Check sheet for the modelled part. Datum: model origin and axes. Units: mm. A direction names the side the tool comes from. Coordinates: 2 decimals unless noted, no trailing zeros. Loops run counter-clockwise (first coordinate to the right, second up) from the corner with the lowest first, then second, coordinate; pieces in that order, holes last. Notation, with made-up numbers: (8, -30) - (64, -30) arc R31 cw to (64, 7) - close; hole circle Ø2 at (-23.75, 36). An arc over 180 degrees is marked (long way). Write each question's results on one line, items separated by ' | '. Start each with the question number.
1. Thickness scan on line 1 (Y direction, x = 0, z = -0.5) (3 decimals); line 2 (Y direction, x = -21.5, z = 0); line 3 (X direction, y = -12.5, z = -0.1). Record the ranges inside material, lowest first. Write a range as [from, to].
2. Cross-section at A-A (x = 0). Record the cut outline in (y, z) (3 decimals), and give its area (3 significant figures).
3. Tool access check on faces 5 (the face through (29.563, 7.238, 0.268)), 6 (the face through (16.02, -25.88, 0.27)), 7 (the face through (-20.35, -15.655, 0.268)). Record the directions out of +Z, -Z, +X, -X, +Y, -Y that give a thin tool (end or side, any length) a straight path to the whole face; none if there is none.
4. Cross-section at D-D (y = -13). Record the cut outline in (x, z), and give its area (3 significant figures).
5. Cross-section at C-C (y = 0). Record the cut outline in (x, z) (3 decimals), and give its area (3 significant figures).
6. Cross-section at B-B (z = 1.05). Record the cut outline in (x, y) (3 decimals).
7. Draft check along Y on faces 1 (the face through (2, 1, 0)), 2 (the face through (-27.469, -12.837, 0.268)), 3 (the face through (-19.66, -23.23, 0.27)), 4 (the face through (-11.646, 32.475, 0.268)). Enter one of: released by +Y, released by -Y, zero draft, split by the parting line, or undercut.
8. Gauge pin test, flat end, axial feed: P1, Ø2.5, axis at x = -0.5, y = -1, coming from the -Z side. Record the tip position at first contact, or that the pin passes through.
```python
from build123d import *

# Parameters (mm, degrees)
BOSS_EXTRUDE1_DEPTH = 1.5
SKETCH2_R           = 4.075
BOSS_EXTRUDE2_DEPTH = 1
SKETCH3_R           = 2
CUT_EXTRUDE1_DEPTH  = 2.5


with BuildPart() as part:
    # Sketch1 → Boss-Extrude1 (new body)
    with BuildSketch(Plane.XY):
        with BuildLine():
            Line((-23.460220375, 25.295613453), (-18.010816917, 19.106590755))
            Line((-18.010816917, 19.106590755), (-24.257098112, 10.052090702))
            Line((-24.257098112, 10.052090702), (-31.977876551, 12.948567925))
            ThreePointArc((-31.977876551, 12.948567925), (-34.489701397, -0.842910146), (-31.307164796, -14.495221021))
            Line((-31.307164796, -14.495221021), (-23.737096152, -11.225043545))
            Line((-23.737096152, -11.225043545), (-17.055961915, -19.96360437))
            Line((-17.055961915, -19.96360437), (-22.1965272, -26.411440329))
            ThreePointArc((-22.1965272, -26.411440329), (-9.856248675, -33.062128819), (4.11132844, -34.254152718))
            Line((4.11132844, -34.254152718), (3.340484701, -26.044049191))
            Line((3.340484701, -26.044049191), (13.715933938, -22.39027674))
            Line((13.715933938, -22.39027674), (18.259668309, -29.27173574))
            ThreePointArc((18.259668309, -29.27173574), (28.398204714, -19.590609204), (33.84810551, -6.675009615))
            Line((33.84810551, -6.675009615), (25.801629236, -4.87106406))
            Line((25.801629236, -4.87106406), (25.532875276, 6.125652327))
            Line((25.532875276, 6.125652327), (33.481622838, 8.320512732))
            ThreePointArc((33.481622838, 8.320512732), (27.407304408, 20.95446647), (16.80795122, 30.128769901))
            Line((16.80795122, 30.128769901), (12.605799132, 23.03356604))
            Line((12.605799132, 23.03356604), (2.064250813, 26.176138082))
            Line((2.064250813, 26.176138082), (2.433112603, 34.414095412))
            ThreePointArc((2.433112603, 34.414095412), (-11.45955905, 32.541181699), (-23.460220375, 25.295613453))
        make_face()
    extrude(amount=BOSS_EXTRUDE1_DEPTH)

    # Sketch2 → Boss-Extrude2 (add)
    with BuildSketch(Plane(origin=(0, 0, 0), x_dir=(-1, 0, 0), z_dir=(0, 0, -1))):
        with BuildLine():
            Line((-2.433112603, 34.414095412), (-2.064250813, 26.176138082))
            Line((-2.064250813, 26.176138082), (-12.605799132, 23.03356604))
            Line((-12.605799132, 23.03356604), (-16.80795122, 30.128769901))
            ThreePointArc((-16.80795122, 30.128769901), (-27.407304408, 20.95446647), (-33.481622838, 8.320512732))
            Line((-33.481622838, 8.320512732), (-25.532875276, 6.125652327))
            Line((-25.532875276, 6.125652327), (-25.801629236, -4.87106406))
            Line((-25.801629236, -4.87106406), (-33.84810551, -6.675009615))
            ThreePointArc((-33.84810551, -6.675009615), (-28.398204714, -19.590609204), (-18.259668309, -29.27173574))
            Line((-18.259668309, -29.27173574), (-13.715933938, -22.39027674))
            Line((-13.715933938, -22.39027674), (-3.340484701, -26.044049191))
            Line((-3.340484701, -26.044049191), (-4.11132844, -34.254152718))
            ThreePointArc((-4.11132844, -34.254152718), (9.856248675, -33.062128819), (22.1965272, -26.411440329))
            Line((22.1965272, -26.411440329), (17.055961915, -19.96360437))
            Line((17.055961915, -19.96360437), (23.737096152, -11.225043545))
            Line((23.737096152, -11.225043545), (31.307164796, -14.495221021))
            ThreePointArc((31.307164796, -14.495221021), (34.489701397, -0.842910146), (31.977876551, 12.948567925))
            Line((31.977876551, 12.948567925), (24.257098112, 10.052090702))
            Line((24.257098112, 10.052090702), (18.010816917, 19.106590755))
            Line((18.010816917, 19.106590755), (23.460220375, 25.295613453))
            ThreePointArc((23.460220375, 25.295613453), (11.45955905, 32.541181699), (-2.433112603, 34.414095412))
        make_face()
        Circle(SKETCH2_R, mode=Mode.SUBTRACT)
    extrude(amount=BOSS_EXTRUDE2_DEPTH)

    # Sketch3 → Cut-Extrude1 (cut, through all)
    with BuildSketch(Plane(origin=(0, 0, 0), x_dir=(-1, 0, 0), z_dir=(0, 0, -1))):
        Circle(SKETCH3_R)
    extrude(amount=-CUT_EXTRUDE1_DEPTH, mode=Mode.SUBTRACT)


solid = part.part
```
Established:
1) line 1: [-34.5, -4.075], [4.075, 34.5] | line 2: [-26.98, -25.54], [-14.15, 14.05], [23.07, 26.98] | line 3: [-32.16, -26.69], [-22.76, 32.16]
2) outline: (-34.5, -1) - (-4.075, -1) - (-4.075, 0) - (-2, 0) - (-2, 1.5) - (-34.5, 1.5) - close; (2, 0) - (4.075, 0) - (4.075, -1) - (34.5, -1) - (34.5, 1.5) - (2, 1.5) - close | area: 158 mm^2
3) face 5: +Z, -Z, +X | face 6: +Z, -Z, -Y | face 7: +Z, -Z
4) outline: (-31.96, -1) - (-27.85, -1) - (-27.85, 1.5) - (-31.96, 1.5) - close; (-22.38, -1) - (31.96, -1) - (31.96, 1.5) - (-22.38, 1.5) - close | area: 146 mm^2
5) outline: (-34.5, -1) - (-4.075, -1) - (-4.075, 0) - (-2, 0) - (-2, 1.5) - (-34.5, 1.5) - close; (2, 0) - (4.075, 0) - (4.075, -1) - (25.683, -1) - (25.683, 1.5) - (2, 1.5) - close | area: 136 mm^2
6) outline: (-31.978, 12.949) arc R34.5 ccw to (-31.307, -14.495) - (-23.737, -11.225) - (-17.056, -19.964) - (-22.197, -26.411) arc R34.5 ccw to (4.111, -34.254) - (3.34, -26.044) - (13.716, -22.39) - (18.26, -29.272) arc R34.5 ccw to (33.848, -6.675) - (25.802, -4.871) - (25.533, 6.126) - (33.482, 8.321) arc R34.5 ccw to (16.808, 30.129) - (12.606, 23.034) - (2.064, 26.176) - (2.433, 34.414) arc R34.5 ccw to (-23.46, 25.296) - (-18.011, 19.107) - (-24.257, 10.052) - close; hole circle Ø4 at (0, 0)
7) face 1: undercut | face 2: released by -Y | face 3: undercut | face 4: released by +Y
8) P1: z = 0
